Geometry check sheet. Reference: the model listing, model coordinates, mm. A direction names the side the tool comes from. Coordinates: 2 decimals unless noted, no trailing zeros. Write each loop counter-clockwise with the first axis right and the second up, starting at its lowest first coordinate (ties: lowest second). Pieces come first, ordered by that corner, then holes. Notation, with made-up numbers: M -9.75,-19.5 L 34.25,-19.5 A25 ccw 34.25,-1.5 Z; hole C -37.5,70.25 d5. An arc over 180 degrees is marked long. Put each result on its own line as item: value. Start each with the question number.
1) Gauge pin test, flat ends, axial feed: pin 1 (5 mm diameter, centred on y = 26, z = 5.5, fed in from -X); pin 2 (1.5 mm diameter, centred on x = -24, z = 3.5, fed in from +Y); pin 3 (1.5 mm diameter, centred on x = -56.5, z = 5, fed in from -Y). Record the tip position at first contact, or that the pin passes through.
2) Cross-section at A-A on x = 0. Record the cut outline in (y, z).
3) Cross-section at B-B on y = 0. Count the separate pieces of the cut face and the enclosed holes in it, plus the area to 3 significant figures.
4) Cross-section at D-D on y = 50. Record the cut outline in (x, z).
5) Scan lines: line 1 along Y through (x, z) = (-2, 3); line 2 along X through (y, z) = (-43.5, 7); line 3 along Y through (x, z) = (0.5, 7.5). Record each from-to range of solid material in increasing order.
6) Mould release check, pull along Y, two halves, no side actions. Record for faces 1 (the cylindrical face through (-3.501, -15.766, 4.93)), 2 (the cylindrical face through (62, 19.52, 4.93)), 3 (the flat face through (0, -20, 5)), 4 (the flat face through (14, -14, 0)): released by +Y, released by -Y, zero draft, split by the parting line, or undercut.
7) Set-up check for faces 5 (the flat face through (-58, 1.5, 5)), 6 (the flat face through (14, -14, 10)): record each of +Z, -Z, +X, -X, +Y, -Y from which the full face is reachable in a straight line by a thin tool's end or side.
from build123d import *

# Parameters (mm, degrees)
SKETCH1_R           = 65
SKETCH1_R_2         = 2.5
SKETCH1_R_3         = 16.15
SKETCH1_R_4         = 4
SKETCH1_R_5         = 1.5
SKETCH1_W           = 50.2
SKETCH1_H           = 10.2
BOSS_EXTRUDE1_DEPTH = 10


with BuildPart() as part:
    # Sketch1 → Boss-Extrude1 (new body)
    with BuildSketch(Plane.XY):
        Circle(SKETCH1_R)
        with Locations((-37.5, 0)):
            Circle(SKETCH1_R_2, mode=Mode.SUBTRACT)
        with Locations((37.5, 0)):
            Circle(SKETCH1_R_2, mode=Mode.SUBTRACT)
        with Locations((0, 50)):
            Circle(SKETCH1_R_2, mode=Mode.SUBTRACT)
        with Locations((0, -50)):
            Circle(SKETCH1_R_2, mode=Mode.SUBTRACT)
        Circle(SKETCH1_R_3, mode=Mode.SUBTRACT)
        with Locations((-41.365746699, 41.365746699)):
            Circle(SKETCH1_R_4, mode=Mode.SUBTRACT)
        with Locations((41.365746699, -41.365746699)):
            Circle(SKETCH1_R_4, mode=Mode.SUBTRACT)
        with Locations((41.365746699, 41.365746699)):
            Circle(SKETCH1_R_4, mode=Mode.SUBTRACT)
        with Locations((-41.365746699, -41.365746699)):
            Circle(SKETCH1_R_4, mode=Mode.SUBTRACT)
        with Locations((48, 0)):
            Circle(SKETCH1_R_5, mode=Mode.SUBTRACT)
        with Locations((58, 0)):
            Circle(SKETCH1_R_5, mode=Mode.SUBTRACT)
        with Locations((-48, 0)):
            Circle(SKETCH1_R_5, mode=Mode.SUBTRACT)
        with Locations((0, -25.1)):
            Rectangle(SKETCH1_W, SKETCH1_H, mode=Mode.SUBTRACT)
        with BuildLine():
            Line((-55.056563459, -1.5), (-60.056563459, -1.5))
            ThreePointArc((-60.056563459, -1.5), (-61.556563459, 0), (-60.056563459, 1.5))
            Line((-60.056563459, 1.5), (-55.056563459, 1.5))
            ThreePointArc((-55.056563459, 1.5), (-53.556563459, 0), (-55.056563459, -1.5))
        make_face(mode=Mode.SUBTRACT)
        with Locations((0, 25.1)):
            Rectangle(SKETCH1_W, SKETCH1_H, mode=Mode.SUBTRACT)
    extrude(amount=BOSS_EXTRUDE1_DEPTH)


solid = part.part
Answer key:
1. pin 1: stops at x = -60.6
1. pin 2: stops at y = 60.7
1. pin 3: stops at y = -33.42
2. outline: M -65,0 L -52.5,0 L -52.5,10 L -65,10 Z; M -47.5,0 L -30.2,0 L -30.2,10 L -47.5,10 Z; M -20,0 L -16.15,0 L -16.15,10 L -20,10 Z; M 16.15,0 L 20,0 L 20,10 L 16.15,10 Z; M 30.2,0 L 47.5,0 L 47.5,10 L 30.2,10 Z; M 52.5,0 L 65,0 L 65,10 L 52.5,10 Z
3. separate pieces: 8
3. enclosed holes: 0
3. area: 707 mm²
4. outline: M -41.53,0 L -2.5,0 L -2.5,10 L -41.53,10 Z; M 2.5,0 L 41.53,0 L 41.53,10 L 2.5,10 Z
5. line 1: y = -64.97 to -51.5, -48.5 to -30.2, -20 to -16.03, 16.03 to 20, 30.2 to 48.5, 51.5 to 64.97
5. line 2: x = -48.3 to -44.75, -37.98 to 37.98, 44.75 to 48.3
5. line 3: y = -65 to -52.45, -47.55 to -30.2, -20 to -16.14, 16.14 to 20, 30.2 to 47.55, 52.45 to 65
6. face 1: undercut
6. face 2: split by the parting line
6. face 3: undercut
6. face 4: zero draft
7. face 5: +Z, -Z
7. face 6: +Z, +X, -X, +Y, -Y
